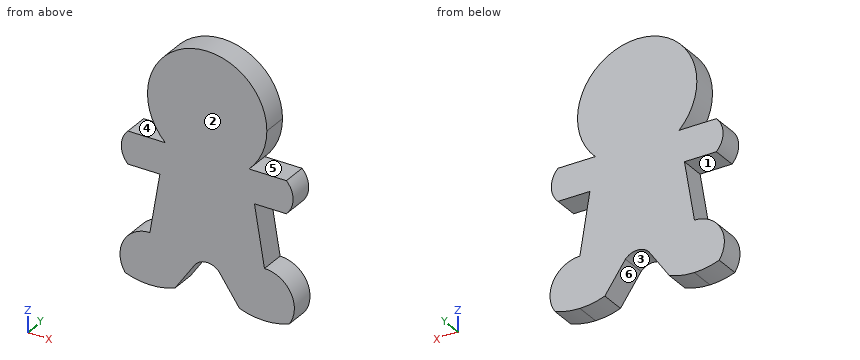
from build123d import *

# Parameters (mm, degrees)
F1_DEPTH = 2.54


with BuildPart() as f1:
    # F0 (on Front) → F1 (new body)
    with BuildSketch(Plane.XZ):
        with BuildLine():
            ThreePointArc((4.2795464076, -4.3412784459), (5.6235811944, -2.3529875795), (6.096, 0))
            ThreePointArc((6.096, 0), (-2.3529875795, 5.6235811944), (-4.2795464076, -4.3412784459))
            Line((-4.2795464076, -4.3412784459), (-3.556, 0))
            Line((-3.556, 0), (0, 0))
            Line((0, 0), (3.556, 0))
            Line((3.556, 0), (4.2795464076, -4.3412784459))
        make_face()
        with BuildLine():
            Line((-3.556, 0), (-4.2795464076, -4.3412784459))
            ThreePointArc((-4.2795464076, -4.3412784459), (0, -6.096), (4.2795464076, -4.3412784459))
            Line((4.2795464076, -4.3412784459), (3.556, 0))
            Line((3.556, 0), (0, 0))
            Line((0, 0), (-3.556, 0))
        make_face()
        with BuildLine():
            ThreePointArc((4.2795464076, -4.3412784459), (0, -6.096), (-4.2795464076, -4.3412784459))
            Line((-4.2795464076, -4.3412784459), (-4.572, -6.096))
            Line((-4.572, -6.096), (-4.829879741, -7.6432784459))
            Line((-4.829879741, -7.6432784459), (-5.8526538527, -13.7799231159))
            Line((-5.8526538527, -13.7799231159), (0, -13.7799231159))
            Line((0, -13.7799231159), (5.8526538527, -13.7799231159))
            Line((5.8526538527, -13.7799231159), (4.829879741, -7.6432784459))
            Line((4.829879741, -7.6432784459), (4.572, -6.096))
            Line((4.572, -6.096), (4.2795464076, -4.3412784459))
        make_face()
        with BuildLine():
            Line((-4.572, -6.096), (-4.2795464076, -4.3412784459))
            Line((-4.2795464076, -4.3412784459), (-8.0895464076, -4.3412784459))
            ThreePointArc((-8.0895464076, -4.3412784459), (-8.7753464076, -5.9922784459), (-8.0895464076, -7.6432784459))
            Line((-8.0895464076, -7.6432784459), (-4.829879741, -7.6432784459))
            Line((-4.829879741, -7.6432784459), (-4.572, -6.096))
        make_face()
        with BuildLine():
            Line((8.0895464076, -4.3412784459), (4.2795464076, -4.3412784459))
            Line((4.2795464076, -4.3412784459), (4.572, -6.096))
            Line((4.572, -6.096), (4.829879741, -7.6432784459))
            Line((4.829879741, -7.6432784459), (8.0895464076, -7.6432784459))
            ThreePointArc((8.0895464076, -7.6432784459), (8.7753464076, -5.9922784459), (8.0895464076, -4.3412784459))
        make_face()
        with BuildLine():
            Line((0, -13.7799231159), (-5.8526538527, -13.7799231159))
            ThreePointArc((-5.8526538527, -13.7799231159), (-8.5487143204, -15.4006894585), (-8.382, -18.542))
            Line((-8.382, -18.542), (-5.842, -18.542))
            Line((-5.842, -18.542), (-3.302, -18.542))
            Line((-3.302, -18.542), (-1.1988751223, -15.5089163039))
            Line((-1.1988751223, -15.5089163039), (0, -13.7799231159))
        make_face()
        with BuildLine():
            ThreePointArc((8.382, -18.542), (8.5487143204, -15.4006894585), (5.8526538527, -13.7799231159))
            Line((5.8526538527, -13.7799231159), (0, -13.7799231159))
            Line((0, -13.7799231159), (1.1988751223, -15.5089163039))
            Line((1.1988751223, -15.5089163039), (3.302, -18.542))
            Line((3.302, -18.542), (5.842, -18.542))
            Line((5.842, -18.542), (8.382, -18.542))
        make_face()
        with BuildLine():
            Line((1.1988751223, -15.5089163039), (0, -13.7799231159))
            Line((0, -13.7799231159), (-1.1988751223, -15.5089163039))
            ThreePointArc((-1.1988751223, -15.5089163039), (0, -14.9736905706), (1.1988751223, -15.5089163039))
        make_face()
        with BuildLine():
            Line((-5.842, -18.542), (-8.382, -18.542))
            ThreePointArc((-8.382, -18.542), (-7.1324099969, -18.8839888715), (-5.842, -18.9992))
            Line((-5.842, -18.9992), (-5.842, -18.542))
        make_face()
        with BuildLine():
            ThreePointArc((5.842, -18.9992), (7.1324099969, -18.8839888715), (8.382, -18.542))
            Line((8.382, -18.542), (5.842, -18.542))
            Line((5.842, -18.542), (5.842, -18.9992))
        make_face()
        with BuildLine():
            Line((-3.302, -18.542), (-5.842, -18.542))
            Line((-5.842, -18.542), (-5.842, -18.9992))
            ThreePointArc((-5.842, -18.9992), (-4.5515900031, -18.8839888715), (-3.302, -18.542))
        make_face()
        with BuildLine():
            Line((5.842, -18.9992), (5.842, -18.542))
            Line((5.842, -18.542), (3.302, -18.542))
            ThreePointArc((3.302, -18.542), (4.5515900031, -18.8839888715), (5.842, -18.9992))
        make_face()
    extrude(amount=F1_DEPTH)


solid = f1.part
Part model, mm, in its own coordinate system. Face numbers are marked on the shaded views. A direction names the side the tool comes from. Give positions to 0.01 mm unless a question says otherwise; leave off trailing zeros. Loops run counter-clockwise (first coordinate to the right, second up) from the corner with the lowest first, then second, coordinate; pieces in that order, holes last. Notation, with made-up numbers: M -27,-12 L 10,-12 A22 cw 10,8 Z; hole C 9.5,-13 d7. An arc over 180 degrees is marked long. Put each result on its own line as item: value. Start each with the question number.
1) Flat gauge pins, fed straight in: pin 1 (1.3 mm diameter, centred on x = -5, y = -1.5, fed in from +Z); pin 2 (0.8 mm diameter, centred on x = 6, y = -2, fed in from +Z); pin 3 (1.3 mm diameter, centred on x = 7, y = -1.5, fed in from -Z). Where does each tip first touch, or does it go through?
2) Saw through at D-D (x = 0). List the corners of the cut face in (y, z).
3) Saw through at B-B (x = -7.5). List the corners of the cut face in (y, z).
4) Saw through at C-C (y = -0.4). List the corners of the cut face in (x, z).
5) Pull direction Z, two halves, no side cores. Call the marked faces 1, 2 and 3: +Z half, -Z half, draft (parallel to the pull), parting line (faces both ways), or undercut.
6) Saw through at A-A (z = -16). List the corners of the cut face in (x, y).
7) Probe probe 1 along Z at (x, y) = (7.5, -0.9); probe 2 along X at (y, z) = (-1.45, -17); probe 3 along Z at (x, y) = (2, -1.85). List the from-to ranges inside material, lowest first.
8) 3-axis set-ups, long thin cutter, end or side, ignore diameter. For the marked faces 4, 5 and 6: which of +Z, -Z, +X, -X, +Y, -Y reach the whole face in a straight line?
Numbers:
1. pin 1: z = 4.27
1. pin 2: z = 2.41
1. pin 3: z = -18.98
2. outline: M -2.54,-14.97 L 0,-14.97 L 0,6.1 L -2.54,6.1 Z
3. outline: M -2.54,-18.81 L 0,-18.81 L 0,-14.26 L -2.54,-14.26 Z; M -2.54,-7.64 L 0,-7.64 L 0,-4.34 L -2.54,-4.34 Z
4. outline: M -8.38,-18.54 A7.28 ccw -3.3,-18.54 L -1.2,-15.51 A1.61 cw 1.2,-15.51 L 3.3,-18.54 A7.28 ccw 8.38,-18.54 A3.05 ccw 5.85,-13.78 L 4.83,-7.64 L 8.09,-7.64 A2.33 ccw 8.09,-4.34 L 4.28,-4.34 A6.1 ccw long -4.28,-4.34 L -8.09,-4.34 A2.33 ccw -8.09,-7.64 L -4.83,-7.64 L -5.85,-13.78 A3.05 ccw Z
5. face 1: undercut
5. face 2: draft
5. face 3: -Z half
6. outline: M -8.79,-2.54 L -1.54,-2.54 L -1.54,0 L -8.79,0 Z; M 1.54,-2.54 L 8.79,-2.54 L 8.79,0 L 1.54,0 Z
7. probe 1: -18.81 to -14.26, -7.64 to -4.34
7. probe 2: -8.9 to -2.23, 2.23 to 8.9
7. probe 3: -16.66 to 5.76
8. face 4: -X, +Y, -Y
8. face 5: +X, +Y, -Y
8. face 6: -Z, +Y, -Y
